Geometry check sheet. Reference: the model listing, model coordinates, mm. Face numbers are marked on the shaded views. A direction names the side the tool comes from. Coordinates: 2 decimals unless noted, no trailing zeros. Loops run counter-clockwise (first coordinate to the right, second up) from the corner with the lowest first, then second, coordinate; pieces in that order, holes last. Notation, with made-up numbers: (62.25, 58.25) - (75.25, 58.25) arc R19 ccw to (75.25, 84.25) - close; hole circle Ø3 at (50.5, 86). An arc over 180 degrees is marked (long way). One line per item, written item: value.
from build123d import *

# Parameters (mm, degrees)
BOSS_EXTRUDE1_DEPTH = 25.4
BOSS_EXTRUDE2_DEPTH = 381
SKETCH3_R           = 36.353481393
CUT_EXTRUDE1_DEPTH  = 381


with BuildPart() as part:
    # Sketch1 → Boss-Extrude1 (new body)
    with BuildSketch(Plane(origin=(0, 0, 0), x_dir=(1, 0, 0), z_dir=(0, 1, 0))):
        Polygon((0, 0), (264.960965784, -150.660965784), (150.660965784, 264.960965784), align=None)
    extrude(amount=BOSS_EXTRUDE1_DEPTH)

    # Sketch2 → Boss-Extrude2 (add)
    with BuildSketch(Plane(origin=(0, 25.4, 0), x_dir=(1, 0, 0), z_dir=(0, 1, 0))):
        Polygon((150.660965784, 264.960965784), (102.937728624, 181.032159524), (181.032159524, -102.937728624), (264.960965784, -150.660965784), align=None)
    extrude(amount=-BOSS_EXTRUDE2_DEPTH)

    # Sketch3 → Cut-Extrude1 (cut)
    with BuildSketch(Plane(origin=(141.984944074, 0, -39.04721545), x_dir=(0.26516504294494564, 0, 0.9642030387838472), z_dir=(-0.9642030387838472, 0, 0.26516504294494564))):
        with Locations((0, -70.290841781)):
            Circle(SKETCH3_R)
        with Locations((0, -173.124599598)):
            Circle(SKETCH3_R)
        with Locations((0, -275.958357416)):
            Circle(SKETCH3_R)
    extrude(amount=-CUT_EXTRUDE1_DEPTH, mode=Mode.SUBTRACT)


solid = part.part
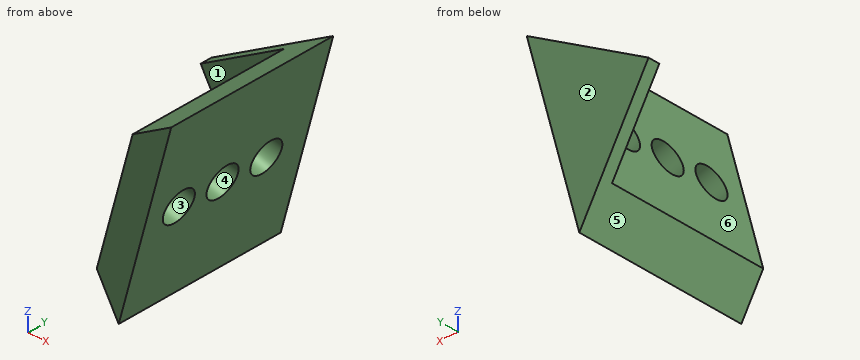
(1) Cross-section at D-D on x = 56. Record the cut outline in (y, z), and give its area (3 significant figures).
Reply:
outline: (0, -98.48) - (25.4, -98.48) - (25.4, 31.84) - (0, 31.84) - close
area: 3,310 mm2
(2) Release check for a two-part mould opening along Z. For the marked faces 3, 4, 5 and 6 record: pulls with the +Z half, pulls with the -Z half, needs draft (parallel to the pull), parting line crosses it, or undercut.
Reply:
face 3: undercut
face 4: undercut
face 5: pulls with the -Z half
face 6: pulls with the +Z half
(3) Go/stop test with flat-tipped pins: pin 1 Ø5 at (y, z) = (-72, 76) entering from +X; pin 2 Ø12 at (y, z) = (-198.5, -162) entering from +X; pin 3 Ø2 at (y, z) = (-123, -77) entering from -X. Record where each tip stops, or that it passes through.
Reply:
pin 1: x = 245.12
pin 2: x = 180.63
pin 3: x = 131.27
(4) Cross-section at A-A on y = -196. Record the cut outline in (x, z), and give its area (3 significant figures).
Reply:
outline: (102.94, -181.03) - (150.66, -264.96) - (200.32, -84.39) - (134.49, -66.29) - close; (149.48, -11.8) - (215.3, -29.91) - (264.96, 150.66) - (181.03, 102.94) - close
area: 20,900 mm2
(5) Access from +Z, -Z, +X, -X, +Y, -Y to the whole of each face (thin tool, end or side, straight path). Record for the marked faces 1 and 2.
Reply:
face 1: +Z, -X, -Y
face 2: +Z, -Z, +X, -X, +Y
(6) Material ranges on probe 1 along Y at (x, z) = (53, -12.5); probe 2 along Y at (x, z) = (205, -65); probe 3 along X at (y, z) = (-155, -95), recorded low to high. Write a range as from..to.
Reply:
probe 1: 0..25.4
probe 2: -355.6..-311.35, -240.57..-208.51, -137.73..-105.68, -34.9..25.4
probe 3: 126.6..197.4
(7) Cross-section at B-B on z = -70. State how many separate pieces and enclosed holes the cut face has, and give its area (3 significant figures).
Reply:
separate pieces: 4
enclosed holes: 0
area: 17,700 mm2
